Geometry check sheet. Reference: the model listing, model coordinates, mm. A direction names the side the tool comes from. Round coordinates to 2 decimals unless told otherwise and drop trailing zeros. Loops run counter-clockwise (first coordinate to the right, second up) from the corner with the lowest first, then second, coordinate; pieces in that order, holes last. Notation, with made-up numbers: M 66,81 L 79,81 A14 cw 79,97 Z; hole C 87,11 d7. An arc over 180 degrees is marked long. Write item = value, one per line.
from build123d import *

# Parameters (mm, degrees)
ESQUISSE2_R             = 4.5
ESQUISSE4_R             = 3
ENL_V_MAT_EXTRU_1_DEPTH = 18


with BuildPart() as part:
    # Base-Balayage: sweep along a path in Esquisse3
    with BuildLine(Plane(origin=(0, 0, 0), x_dir=(0, 0, -1), z_dir=(1, 0, 0))) as base_balayage_path:
        Line((0, 0), (-20, 0))
        ThreePointArc((-20, 0), (-29.5, 9.5), (-20, 19))
        Line((-20, 19), (0, 19))
    # Esquisse2 → Base-Balayage (sweep)
    with BuildSketch(Plane.XY):
        Circle(ESQUISSE2_R)
    sweep(path=base_balayage_path.line)

    # Esquisse4 → Enlèv. mat.-Extru.1 (cut)
    with BuildSketch(Plane(origin=(0, 0, 0), x_dir=(-1, 0, 0), z_dir=(0, 0, -1))):
        with Locations(Location((0, 19, 0), (0, 0, 90))):
            Circle(ESQUISSE4_R)
        with Locations(Location((0, 0, 0), (0, 0, 90))):
            Circle(ESQUISSE4_R)
    extrude(amount=-ENL_V_MAT_EXTRU_1_DEPTH, mode=Mode.SUBTRACT)


solid = part.part
(1) Depth check by flat-ended pin: pin 1 Ø3 at (y, z) = (-1.5, 30) entering from +X; pin 2 Ø1.5 at (x, y) = (-0.5, 18) entering from +Z; pin 3 Ø3 at (x, y) = (1, 19) entering from -Z. Enter the tip coordinate at first touch or a pass-through.
Result set:
pin_1 = 2.3
pin_2 = 31.63
pin_3 = 18
(2) Tool access check on faces 4 (the flat face through (-1, 16, 0)), 5 (the flat face through (0, 19, 18)). Record the directions out of +Z, -Z, +X, -X, +Y, -Y that give a thin tool (end or side, any length) a straight path to the whole face; none if there is none.
Result set:
face_4 = -Z, +X, -X, +Y, -Y
face_5 = -Z
(3) Sectioned sample at A-A on z = 16. Record the cut outline in (x, y).
Result set:
outline = C 0,0 d9; C 0,19 d9; hole C 0,0 d6; hole C 0,19 d6
(4) Sectioned sample at C-C on y = 9.5. Record the cut outline in (x, z), then the cut area to 3 significant figures.
Result set:
outline = C 0,29.5 d9
area = 63.6 mm2
(5) Material ranges on line 1 along Y through (x, z) = (0.25, 5.5); line 2 along Y through (x, z) = (-0.75, 12.5); line 3 along X through (y, z) = (19, 6.75), recorded low to high. Write a range as from..to.
Result set:
line_1 = -4.49..-2.99, 2.99..4.49, 14.51..16.01, 21.99..23.49
line_2 = -4.44..-2.9, 2.9..4.44, 14.56..16.1, 21.9..23.44
line_3 = -4.5..-3, 3..4.5
(6) Release check for a two-part mould opening along X. For faces 1 (the cylindrical face through (-0.59, 4.46, 10.14)), 2 (the flat face through (1, -3, 0)), 3 (the cylindrical face through (0.9, 2.86, 8.87)) record: released by +X, released by -X, zero draft, split by the parting line, or undercut.
Result set:
face_1 = split by the parting line
face_2 = zero draft
face_3 = undercut
(7) Sectioned sample at B-B on x = 0. Record the cut outline in (y, z).
Result set:
outline = M -4.5,0 L -3,0 L -3,18 L 3,18 L 3,0 L 4.5,0 L 4.5,20 A5 cw 14.5,20 L 14.5,0 L 16,0 L 16,18 L 22,18 L 22,0 L 23.5,0 L 23.5,20 A14 ccw -4.5,20 Z
